from build123d import *

# Parameters (mm, degrees)
F1_DEPTH = 140
F2_R     = 10
F3_DEPTH = 400.001
F5_DEPTH = 40.001


with BuildPart() as f1:
    # F0 (on Top) → F1 (new body)
    with BuildSketch(Plane.XY):
        with BuildLine():
            Line((202.315605, 14.572916), (-195.684395, 14.572916))
            ThreePointArc((-195.684395, 14.572916), (-196.391502, 14.280022), (-196.684395, 13.572916))
            Line((-196.684395, 13.572916), (-196.684395, -25.427084))
            Line((-196.684395, -25.427084), (-190.684395, -25.427084))
            Line((-190.684395, -25.427084), (-190.684395, 7.572916))
            ThreePointArc((-190.684395, 7.572916), (-190.391502, 8.280022), (-189.684395, 8.572916))
            Line((-189.684395, 8.572916), (196.315605, 8.572916))
            ThreePointArc((196.315605, 8.572916), (197.022712, 8.280022), (197.315605, 7.572916))
            Line((197.315605, 7.572916), (197.315605, -25.427084))
            Line((197.315605, -25.427084), (203.315605, -25.427084))
            Line((203.315605, -25.427084), (203.315605, 13.572916))
            ThreePointArc((203.315605, 13.572916), (203.022712, 14.280022), (202.315605, 14.572916))
        make_face()
    extrude(amount=F1_DEPTH)

    # F2 (on face) → F3 (cut, through all)
    with BuildSketch(Plane.YZ.offset(203.315605)):
        with BuildLine():
            Line((3.824211, 140.531208), (-66.175789, 140.531208))
            Line((-66.175789, 140.531208), (-66.175789, -19.468792))
            Line((-66.175789, -19.468792), (3.824211, -19.468792))
            Line((3.824211, -19.468792), (3.824211, 0))
            Line((3.824211, 0), (-5.427084, 0))
            ThreePointArc((-5.427084, 0), (-19.56922, 5.857864), (-25.427084, 20))
            Line((-25.427084, 20), (-25.427084, 120))
            ThreePointArc((-25.427084, 120), (-19.56922, 134.142136), (-5.427084, 140))
            Line((-5.427084, 140), (3.824211, 140))
            Line((3.824211, 140), (3.824211, 140.531208))
        make_face()
        with Locations((-5.427084, 20)):
            Circle(F2_R)
        with Locations((-5.427084, 120)):
            Circle(F2_R)
    extrude(amount=-F3_DEPTH, mode=Mode.SUBTRACT)

    # F4 (on face) → F5 (cut, through all)
    with BuildSketch(Plane(origin=(0, 14.572916, 0), x_dir=(-1, 0, 0), z_dir=(0, 1, 0))):
        with BuildLine():
            ThreePointArc((-187.315605, 84.966576), (-184.3914, 77.900238), (-177.328978, 74.966585))
            Line((-177.328978, 74.966585), (-15.013373, 74.749518))
            ThreePointArc((-15.013373, 74.749518), (-7.933662, 77.673715), (-5, 84.749509))
            Line((-5, 84.749509), (-5, 120.333677))
            ThreePointArc((-5, 120.333677), (-7.928932, 127.404745), (-15, 130.333677))
            Line((-15, 130.333677), (-177.315605, 130.333677))
            ThreePointArc((-177.315605, 130.333677), (-184.386673, 127.404745), (-187.315605, 120.333677))
            Line((-187.315605, 120.333677), (-187.315605, 84.966576))
        make_face()
        with BuildLine():
            Line((180.684395, 84.50119), (180.684395, 120.333677))
            ThreePointArc((180.684395, 120.333677), (177.755463, 127.404745), (170.684395, 130.333677))
            Line((170.684395, 130.333677), (15, 130.333677))
            ThreePointArc((15, 130.333677), (7.928932, 127.404745), (5, 120.333677))
            Line((5, 120.333677), (5, 84.709389))
            ThreePointArc((5, 84.709389), (7.924206, 77.643051), (14.986627, 74.709398))
            Line((14.986627, 74.709398), (170.671022, 74.501199))
            ThreePointArc((170.671022, 74.501199), (177.750733, 77.425396), (180.684395, 84.50119))
        make_face()
        with BuildLine():
            ThreePointArc((-187.315605, 19.666323), (-184.386673, 12.595255), (-177.315605, 9.666323))
            Line((-177.315605, 9.666323), (-15, 9.666323))
            ThreePointArc((-15, 9.666323), (-7.928932, 12.595255), (-5, 19.666323))
            Line((-5, 19.666323), (-5, 55.250491))
            ThreePointArc((-5, 55.250491), (-7.933662, 62.326285), (-15.013373, 65.250482))
            Line((-15.013373, 65.250482), (-177.328978, 65.033415))
            ThreePointArc((-177.328978, 65.033415), (-184.3914, 62.099762), (-187.315605, 55.033424))
            Line((-187.315605, 55.033424), (-187.315605, 19.666323))
        make_face()
        with BuildLine():
            ThreePointArc((5, 19.666323), (7.928932, 12.595255), (15, 9.666323))
            Line((15, 9.666323), (170.684395, 9.666323))
            ThreePointArc((170.684395, 9.666323), (177.755463, 12.595255), (180.684395, 19.666323))
            Line((180.684395, 19.666323), (180.684395, 55.49881))
            ThreePointArc((180.684395, 55.49881), (177.750733, 62.574604), (170.671022, 65.498801))
            Line((170.671022, 65.498801), (14.986627, 65.290602))
            ThreePointArc((14.986627, 65.290602), (7.924206, 62.356949), (5, 55.290611))
            Line((5, 55.290611), (5, 19.666323))
        make_face()
    extrude(amount=-F5_DEPTH, mode=Mode.SUBTRACT)


solid = f1.part
For this review, take the finished solid that the model builds, in its own axes (mm). A direction names the side the tool comes from. Round coordinates to 2 decimals unless told otherwise and drop trailing zeros. Loops run counter-clockwise (first coordinate to the right, second up) from the corner with the lowest first, then second, coordinate; pieces in that order, holes last. Notation, with made-up numbers: (-36, -11.75) - (-10, -11.75) arc R28 cw to (-10, 24.25) - close; hole circle Ø7 at (33.5, 55). An arc over 180 degrees is marked (long way). Use one line per item in the form item = value.
1) Mouldability with a two-part tool opening along Z and no side actions: class faces 4 (the face through (-177.83, 11.61, 127.33)), 5 (the face through (200.36, -19.41, 5.7)), 6 (the face through (-193.64, -19.72, 133.99)) as pulls with the +Z half, pulls with the -Z half, needs draft (parallel to the pull), parting line crosses it, or undercut.
Solutions:
face_4 = undercut
face_5 = pulls with the -Z half
face_6 = pulls with the +Z half
2) Wall thickness on probe 1 along X at (y, z) = (12, 54); probe 2 along X at (y, z) = (3, 31); probe 3 along Z at (x, y) = (-98, 11): over which ranges is each line inside the solid? List them lowest first.
Solutions:
probe_1 = -196.68 to -180.68, -5 to 5, 187.32 to 203.32
probe_2 = -196.68 to -190.68, 197.32 to 203.32
probe_3 = 0 to 9.67, 65.4 to 74.6, 130.33 to 140
3) Tool access review of faces 1 (the face through (-177.68, 11.61, 12.52)), 2 (the face through (200.36, -19.72, 133.99)), 3 (the face through (-190.684, -9, 69)): name each direction out of +Z, -Z, +X, -X, +Y, -Y from which nothing blocks a thin tool from reaching the whole face with its end or side.
Solutions:
face_1 = +Y, -Y
face_2 = +Z, +X, -X, -Y
face_3 = +Z, -Z, -Y
4) We need section B-B on x = 53. Write out the cut boundary in (y, z).
Solutions:
outline = (8.57, 0) - (14.57, 0) - (14.57, 9.67) - (8.57, 9.67) - close; (8.57, 65.2) - (14.57, 65.2) - (14.57, 74.8) - (8.57, 74.8) - close; (8.57, 130.33) - (14.57, 130.33) - (14.57, 140) - (8.57, 140) - close
5) We need section A-A on z = 37. Write out the cut boundary in (x, y), then the cut area to 3 significant figures.
Solutions:
outline = (-196.68, -25.43) - (-190.68, -25.43) - (-190.68, 7.57) arc R1 cw to (-189.68, 8.57) - (-180.68, 8.57) - (-180.68, 14.57) - (-195.68, 14.57) arc R1 ccw to (-196.68, 13.57) - close; (-5, 8.57) - (5, 8.57) - (5, 14.57) - (-5, 14.57) - close; (187.32, 8.57) - (196.32, 8.57) arc R1 cw to (197.32, 7.57) - (197.32, -25.43) - (203.32, -25.43) - (203.32, 13.57) arc R1 ccw to (202.32, 14.57) - (187.32, 14.57) - close
area = 660 mm2
6) We need section C-C on y = -1. Write out the cut boundary in (x, z).
Solutions:
outline = (-196.68, 0) - (-190.68, 0) - (-190.68, 11.03) - (-196.68, 11.03) - close; (-196.68, 28.97) - (-190.68, 28.97) - (-190.68, 111.03) - (-196.68, 111.03) - close; (-196.68, 128.97) - (-190.68, 128.97) - (-190.68, 140) - (-196.68, 140) - close; (197.32, 0) - (203.32, 0) - (203.32, 11.03) - (197.32, 11.03) - close; (197.32, 28.97) - (203.32, 28.97) - (203.32, 111.03) - (197.32, 111.03) - close; (197.32, 128.97) - (203.32, 128.97) - (203.32, 140) - (197.32, 140) - close
7) Clearance check with a flat-ended pin moving along its axis: P1, Ø5, axis at x = -117.5, y = 10.5, coming from the -Z side. State where the tip first meets the part, or that it passes through.
Solutions:
P1 = 0
8) We need section D-D on z = 16. Write out the cut boundary in (x, y), then the cut area to 3 significant figures.
Solutions:
outline = (-196.68, -25.02) - (-190.68, -25.02) - (-190.68, -14.59) - (-196.68, -14.59) - close; (-196.68, 3.74) - (-190.68, 3.74) - (-190.68, 7.57) arc R1 cw to (-189.68, 8.57) - (-179.99, 8.57) - (-179.99, 14.57) - (-195.68, 14.57) arc R1 ccw to (-196.68, 13.57) - close; (-5.7, 8.57) - (5.7, 8.57) - (5.7, 14.57) - (-5.7, 14.57) - close; (186.62, 8.57) - (196.32, 8.57) arc R1 cw to (197.32, 7.57) - (197.32, 3.74) - (203.32, 3.74) - (203.32, 13.57) arc R1 ccw to (202.32, 14.57) - (186.62, 14.57) - close; (197.32, -25.02) - (203.32, -25.02) - (203.32, -14.59) - (197.32, -14.59) - close
area = 452 mm2
